Drawing for the job (mm, zero at the part's lowest x, y, z). Give positions to 0.01 mm unless a question says otherwise; leave off trailing zeros. Order: outer loops, then holes, each group sorted by start corner. A loop starts at its lowest first (then second) coordinate and runs counter-clockwise, first axis right, second up. Notation, with made-up numbers: M 17,15 L 48,15 A21 ccw 48,35 Z; hole C 58.25,27 d9. An arc over 180 degrees is marked long. One line per item, written item: value.
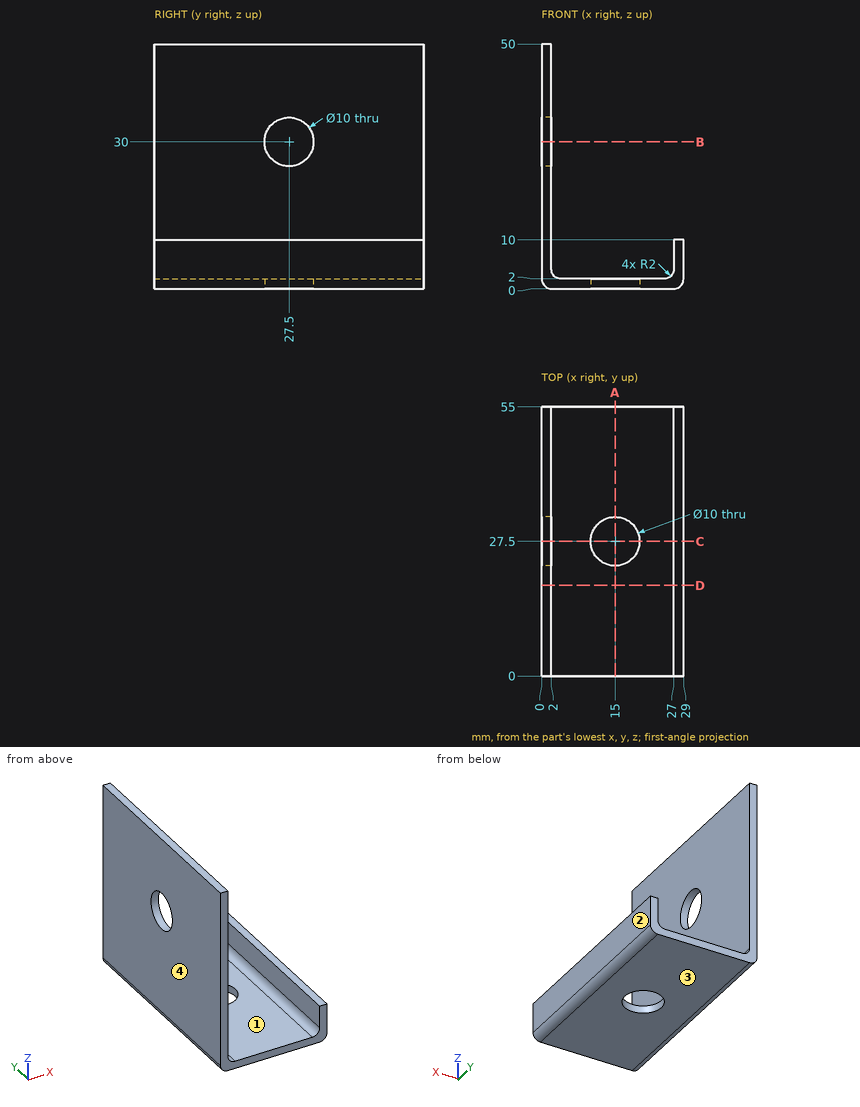
1) Mould opens along X. For the marked faces 1, 2, 3 and 4 say: released by +X, released by -X, zero draft, split by the parting line, or undercut.
Check values:
face 1: undercut
face 2: released by +X
face 3: zero draft
face 4: released by -X
2) Saw through at A-A, the plane x = 15. Write the cut outline in (y, z).
Check values:
outline: M 0,0 L 22.5,0 L 22.5,2 L 0,2 Z; M 32.5,0 L 55,0 L 55,2 L 32.5,2 Z
3) Saw through at C-C, the plane y = 27.5. Write the cut outline in (x, z).
Check values:
outline: M 0,2 A2 ccw 2,0 L 10,0 L 10,2 L 4,2 A2 cw 2,4 L 2,25 L 0,25 Z; M 0,35 L 2,35 L 2,50 L 0,50 Z; M 20,0 L 27,0 A2 ccw 29,2 L 29,10 L 27,10 L 27,4 A2 cw 25,2 L 20,2 Z
4) Saw through at B-B, the plane z = 30. Write the cut outline in (x, y).
Check values:
outline: M 0,0 L 2,0 L 2,22.5 L 0,22.5 Z; M 0,32.5 L 2,32.5 L 2,55 L 0,55 Z
5) Drill centre lines: probe 1 along X at (y, z) = (33, 5.5); probe 2 along Y at (x, z) = (15, 1.4); probe 3 along X at (y, z) = (33, 39). Where is each one in solid material? Low to high. Write a range as from..to.
Check values:
probe 1: 0..2, 27..29
probe 2: 0..22.5, 32.5..55
probe 3: 0..2
6) Saw through at D-D, the plane y = 18.5. Write the cut outline in (x, z), then the cut area to 3 significant figures.
Check values:
outline: M 0,2 A2 ccw 2,0 L 27,0 A2 ccw 29,2 L 29,10 L 27,10 L 27,4 A2 cw 25,2 L 4,2 A2 cw 2,4 L 2,50 L 0,50 Z
area: 170 mm^2
7) Pin check, flat tips, straight feed: pin 1 (1.5 mm diameter, centred on y = 32.5, z = 35, fed in from +X); pin 2 (6 mm diameter, centred on x = 10.5, y = 29, fed in from +Z); pin 3 (17 mm diameter, centred on x = 19.5, y = 22.5, fed in from +Z). Stop position of each tip, or through.
Check values:
pin 1: x = 2
pin 2: z = 2
pin 3: z = 10
